Drawing for the job (mm, zero at the part's lowest x, y, z). Coordinates: 2 decimals unless noted, no trailing zeros. Write each loop counter-clockwise with the first axis right and the second up, starting at its lowest first coordinate (ties: lowest second). Pieces come first, ordered by that corner, then holes. Notation, with made-up numbers: (89.25, 52) -> (103.25, 52) arc R20 cw to (103.25, 59) -> close; hole circle Ø3 at (-37, -18). An arc over 180 degrees is marked (long way). Write each question's results on one line, items separated by ' | '. Start each with the question number.
Q1. Saw through at A-A on z = 1.75. Give the cut face in (x, y) (1 decimal), and give its area (3 significant figures).
Q2. Two-plate mould, pull along Y, no slides. Class the marked faces 1, 2 and 3: released by +Y, released by -Y, zero draft, split by the parting line, or undercut.
Q3. Drop flat-ended pins along their axis: pin 1 Ø1.5 at (x, z) = (14, 1.5) entering from -Y (1 decimal); pin 2 Ø1.5 at (x, y) = (4, 5) entering from -Z; pin 3 Ø1 at (y, z) = (17.5, 2) entering from +X (1 decimal). Give the stop position or say it passes through.
Q4. Drill centre lines: line 1 (Y direction, x = 9.25, z = 1.1) (1 decimal); line 2 (X direction, y = 17, z = 0.35) (1 decimal); line 3 (X direction, y = 11.25, z = 1.25) (1 decimal). Where is each one in solid material? Low to high.
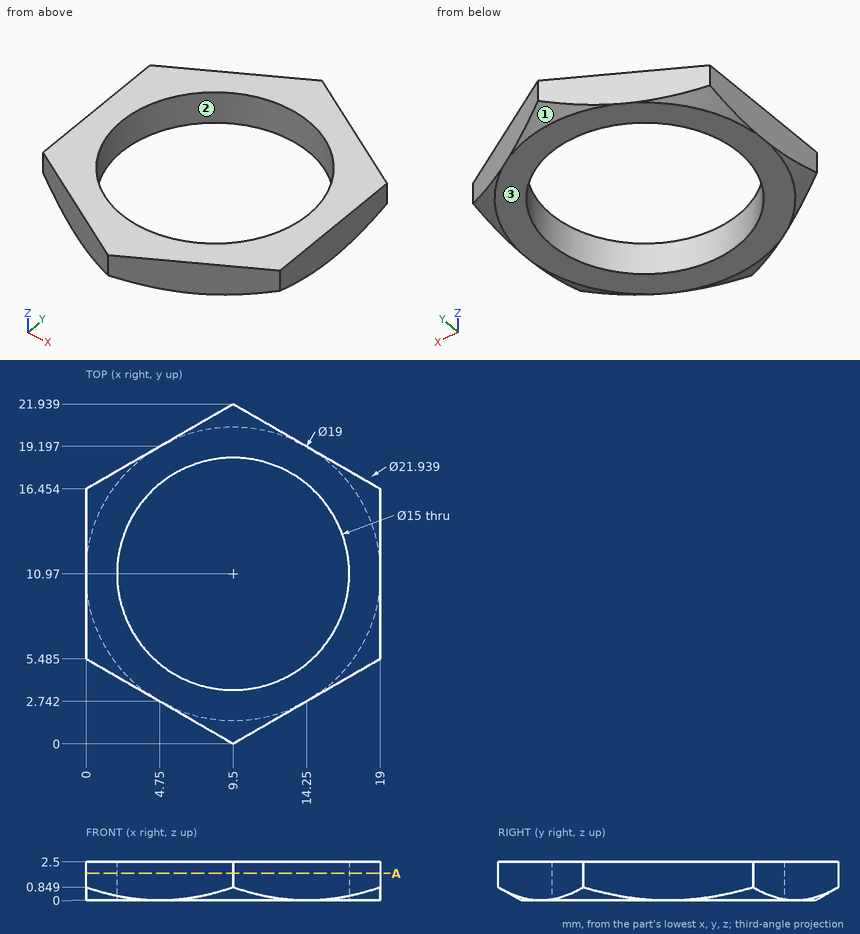
Returned:
1) outline: (0, 5.5) -> (9.5, 0) -> (19, 5.5) -> (19, 16.5) -> (9.5, 21.9) -> (0, 16.5) -> close; hole circle Ø15 at (9.5, 11) | area: 136 mm2
2) face 1: released by +Y | face 2: undercut | face 3: zero draft
3) pin 1: stops at y = 2.2 | pin 2: stops at z = 0 | pin 3: stops at x = 18.1
4) line 1: y = 0.1 to 3.5, 18.5 to 21.8 | line 2: x = 1.4 to 5, 14 to 17.6 | line 3: x = 0 to 2, 17 to 19
